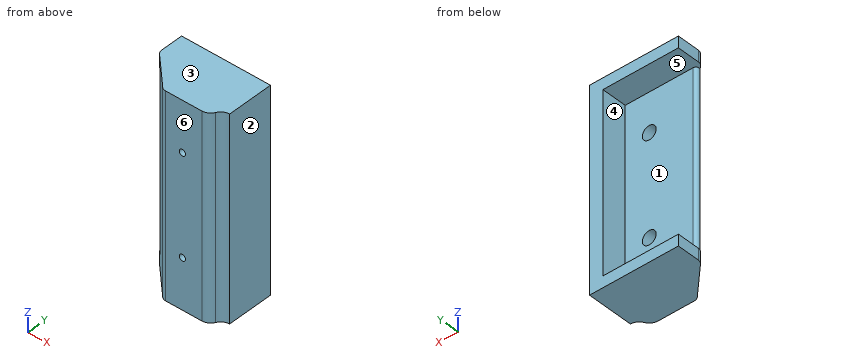
Autodesk Inventor part; units mm, degrees
ref_plane "YZ Plane" through (0, 0, 0) normal (1, 0, 0) x (0, 1, 0)
ref_plane "XZ Plane" through (0, 0, 0) normal (0, 1, 0) x (-1, 0, 0)
ref_plane "XY Plane" through (0, 0, 0) normal (0, 0, 1) x (1, 0, 0)
sketch "Sketch1" plane through (0, 0, 0) normal (0, 0, 1) x (1, 0, 0)
  line L0 (0, 0) -> (58.42, 0)
  line L1 (29.21, 0) -> (29.21, -11.176)
  line L2 (0, 0) -> (29.21, 0)
  line L3 (29.21, 0) -> (29.21, -11.176)
  line L4 (29.21, -11.176) -> (0, -11.176)
  line L5 (0, -11.176) -> (0, 0)
  line L6 (0, -11.176) -> (11.176, -11.176)
  line L7 (11.176, -11.176) -> (0, 0)
  line L8 (59.055, 0) -> (29.21, 0)
  line L9 (29.21, 0) -> (29.21, -11.176)
  line L10 (58.42, 0) -> (29.21, 0)
  line L11 (29.21, 0) -> (29.21, -11.176)
  line L12 (29.21, -11.176) -> (50.4337, -11.176)
  line L13 (58.42, -11.176) -> (58.42, -10.16)
  line L14 (58.42, -11.176) -> (90.1357, -11.176)
  line L15 (90.1357, -11.176) -> (90.1357, 0)
  line L16 (90.1357, 0) -> (68.58, 0)
  line L17 (58.42, 0) -> (58.42, -11.176)
  arc A0 (68.58, 0) -> (59.5068, -5.588) centre (68.58, -10.16) ccw
  arc A1 (50.4337, -11.176) -> (59.5068, -5.588) centre (50.4337, -1.016) ccw
  line L18 (58.42, 0) -> (68.58, 0)
  point P0 (58.42, -7.2964)
  dimension "d1" = 11.176
  dimension "d2" = 11.176
  dimension "d3" = 10.16
  dimension "d6" = 68.58
  dimension "d7" = 10.16
extrude "Extrusion1" add sketch "Sketch1" along normal blind 203.2 contours L0 L1 L4 L7 | L0 L17 A1 L12 L1 | L8 L18 A0 A1 L17
sketch "Sketch2" plane through (0, 0, 203.2) normal (0, 0, 1) x (1, 0, 0)
  line L0 (11.176, -11.176) -> (50.4337, -11.176)
  line L1 (11.176, -11.176) -> (-21.1529, 21.1529)
  line L2 (0, 0) -> (11.176, -11.176)
  line L3 (-21.1529, 21.1529) -> (68.58, 21.1529)
  arc A0 (68.58, 0) -> (59.5068, -5.588) centre (68.58, -10.16) ccw
  line L4 (68.58, 21.1529) -> (68.58, 0)
  arc A1 (57.404, 8.0148) -> (49.5263, -0.5588) centre (68.58, -10.16) ccw
  line L5 (57.404, 8.0148) -> (57.404, 9.9769)
  line L6 (5.8283, 9.9769) -> (19.0786, -3.2734)
  line L7 (31.6162, 9.9769) -> (31.6162, 0)
  line L8 (68.58, 0) -> (0, 0)
  line L9 (26.0282, 9.9769) -> (26.0282, 0)
  line L10 (37.2042, 9.9769) -> (37.2042, 0)
  point P0 (15.8053, 0)
  point P1 (26.0282, 0)
  point P2 (37.2042, 0)
  point P3 (49.8184, 0)
  dimension "d9" = 45.72
  dimension "d11" = 5.588
  dimension "d12" = 5.588
extrude "Extrusion2" add sketch "Sketch2" against normal blind 203.2
sketch "Sketch3" plane through (-21.1529, 21.1529, 203.2) normal (0, 1, 0) x (1, 0, 0)
  line L0 (0, 0) -> (0, 203.2)
  line L1 (0, 101.6) -> (76.2, 101.6)
  line L2 (76.2, 101.6) -> (76.2, 191.77)
  line L3 (76.2, 191.77) -> (76.2, 11.43)
  line L4 (76.2, 191.77) -> (0, 191.77)
  line L5 (0, 191.77) -> (0, 11.43)
  line L6 (0, 11.43) -> (76.2, 11.43)
  line L7 (76.2, 11.43) -> (76.2, 191.77)
  line L8 (89.7329, 0) -> (0, 0)
  line L9 (89.7329, 0) -> (89.7329, 203.2)
  line L10 (0, 203.2) -> (89.7329, 203.2)
  line L11 (0, 0) -> (0, 203.2)
  point P0 (21.1529, 203.2)
  dimension "d15" = 76.2
  dimension "d16" = 90.17
  dimension "d17" = 180.34
extrude "Extrusion3" add sketch "Sketch3" along normal blind 25.4 contours L0 L6 L3 L2 L4 L10 L9 L8
sketch "Sketch4" plane through (-21.1529, 21.1529, 11.43) normal (0, 1, 0) x (1, 0, 0)
  line L0 (32.3289, 11.43) -> (71.5866, 11.43)
  line L1 (71.5866, 11.43) -> (71.5866, -191.77)
  line L2 (32.3289, -191.77) -> (71.5866, -191.77)
  line L3 (32.3289, 11.43) -> (32.3289, -191.77)
  line L4 (32.3289, -90.17) -> (71.5866, -90.17)
  line L5 (51.9578, -90.17) -> (51.9578, 11.43)
  line L6 (51.9578, -90.17) -> (51.9578, -191.77)
  circle A0 centre (51.9578, -140.97) radius 6.985
  circle A1 centre (51.9578, -39.37) radius 6.985
  point P0 (21.1529, 11.43)
  dimension "d20" = 13.97
  dimension "d21" = 13.97
extrude "Extrusion4" cut sketch "Sketch4" against normal blind 19.05 contours A1 L5 | L5 A1 | A0 L6 | L6 A0
fillet "Fillet1" radius 3.175 1 edges at (-21.1529, 21.1529, 101.6)
fillet "Fillet2" radius 6.35 2 edges at (-21.1529, 21.1529, 5.715) (-21.1529, 21.1529, 197.485)
fillet "Fillet3" radius 6.35 1 edges at (11.176, -11.176, 101.6)
sketch "Sketch5" plane through (30.8048, 2.1029, 152.4) normal (0, 1, 0) x (1, 0, 0)
  line L0 (-21.4887, -50.8) -> (-21.4887, 152.4)
  line L1 (-44.2926, -39.37) -> (-44.2926, 140.97)
  line L2 (-44.2926, -39.37) -> (24.2422, -39.37)
  line L3 (24.2422, -39.37) -> (24.2422, 140.97)
  line L4 (24.2422, 140.97) -> (-44.2926, 140.97)
  circle A0 centre (0, 0) radius 6.985
  circle A1 centre (0, 101.6) radius 6.985
  circle A2 centre (0, 101.6) radius 3.175
  circle A3 centre (0, 0) radius 3.175
  point P0 (-30.8048, 152.4)
  dimension "d27" = 6.35
  dimension "d28" = 6.35
extrude "Extrusion5" cut sketch "Sketch5" against normal blind 25.4 contours A2 | A3
properties part number "Battery mount bottom" material "Rubber, Silicone"
Geometry check sheet. Reference: the model listing, model coordinates, mm. Face numbers are marked on the shaded views. A direction names the side the tool comes from. Coordinates: 2 decimals unless noted, no trailing zeros. Write each loop counter-clockwise with the first axis right and the second up, starting at its lowest first coordinate (ties: lowest second). Pieces come first, ordered by that corner, then holes. Notation, with made-up numbers: M 19.5,18 L 38.5,18 A16 cw 38.5,44 Z; hole C -24.5,-2 d1. An arc over 180 degrees is marked long. One line per item, written item: value. Start each with the question number.
(1) Sectioned sample at C-C, the plane z = 175. Enter the section's corners in (x, y) (3 decimals).
(2) Tool access check on the marked faces 1 and 2. Record the directions out of +Z, -Z, +X, -X, +Y, -Y that give a thin tool (end or side, any length) a straight path to the whole face; none if there is none.
(3) Scan lines: line 1 along Z through (x, y) = (27.5, 24); line 2 along X through (y, z) = (35, 51); line 3 along X through (y, z) = (-4.25, 152.4). Record each from-to range of solid material in increasing order. Write a range as [from, to].
(4) Depth check by flat-ended pin: pin 1 (1.5 mm diameter, centred on x = -3.5, z = 24.5, fed in from -Y); pin 2 (20.5 mm diameter, centred on y = 39.5, z = 79, fed in from -X); pin 3 (15.5 mm diameter, centred on x = 34, z = 50, fed in from +Y). Enter the tip coordinate at first touch or a pass-through.
(5) Sectioned sample at D-D, the plane x = 57.5. Enter the section's corners in (y, z), and give its area (3 significant figures).
(6) Sectioned sample at A-A, the plane y = 32.5. Enter the section's corners in (x, z).
(7) Release check for a two-part mould opening along Z. For the marked faces 3, 4, 5 and 6 record: released by +Z, released by -Z, zero draft, split by the parting line, or undercut.
(8) Sectioned sample at B-B, the plane z = 152.4. Enter the section's corners in (x, y) (3 decimals).
Filled sheet:
1. outline: M -15.733,15.733 L 9.316,-9.316 A6.35 ccw 13.806,-11.176 L 50.434,-11.176 A10.16 ccw 59.507,-5.588 A10.16 cw 68.58,0 L 68.58,46.553 L 55.047,46.553 L 55.047,21.153 L -13.488,21.153 A3.175 ccw Z
2. face 1: -X, +Y
2. face 2: +Z, -Z, +X, +Y, -Y
3. line 1: [0, 11.43], [191.77, 203.2]
3. line 2: [55.05, 68.58]
3. line 3: [4.25, 27.63], [33.98, 60.32]
4. pin 1: y = 2.75
4. pin 2: x = 55.05
4. pin 3: y = 21.15
5. outline: M -8.32,0 L 46.55,0 L 46.55,203.2 L -8.32,203.2 Z
5. area: 11,100 mm²
6. outline: M -21.15,0 L 68.58,0 L 68.58,203.2 L -21.15,203.2 L -21.15,191.77 L 55.05,191.77 L 55.05,11.43 L -21.15,11.43 Z
7. face 3: released by +Z
7. face 4: undercut
7. face 5: undercut
7. face 6: zero draft
8. outline: M -15.733,15.733 L 9.316,-9.316 A6.35 ccw 13.806,-11.176 L 27.63,-11.176 L 27.63,2.103 L 23.82,2.103 L 23.82,21.153 L -13.488,21.153 A3.175 ccw Z; M 33.98,-11.176 L 50.434,-11.176 A10.16 ccw 59.507,-5.588 A10.16 cw 68.58,0 L 68.58,46.553 L 55.047,46.553 L 55.047,21.153 L 37.79,21.153 L 37.79,2.103 L 33.98,2.103 Z
